Part model, mm, in its own coordinate system. A direction names the side the tool comes from. Round coordinates to 2 decimals unless told otherwise and drop trailing zeros. Write each loop counter-clockwise with the first axis right and the second up, starting at its lowest first coordinate (ties: lowest second). Pieces come first, ordered by that corner, then holes.
```python
from build123d import *

# Parameters (mm, degrees)
F1_DEPTH = 12.7
F3_DEPTH = 21.336
F6_D     = 4.7625
F6_DEPTH = 3.175
F6_TIP   = 1.4307993491
F7_W     = 6.096
F7_H     = 22.606
F7_W_2   = 22.606
F7_H_2   = 6.096
F8_DEPTH = 2.54
F9_DEPTH = 2.54


with BuildPart() as f1:
    # F0 (on Top) → F1 (new body)
    with BuildSketch(Plane.XY):
        with BuildLine():
            Line((40.4105676174, 15.0449029118), (15.0105676174, 15.0449029118))
            ThreePointArc((15.0105676174, 15.0449029118), (10.5204395569, 13.1850309723), (8.6605676174, 8.6949029118))
            Line((8.6605676174, 8.6949029118), (8.6605676174, -16.7050970882))
            ThreePointArc((8.6605676174, -16.7050970882), (10.5204395569, -21.1952251488), (15.0105676174, -23.0550970882))
            Line((15.0105676174, -23.0550970882), (40.4105676174, -23.0550970882))
            ThreePointArc((40.4105676174, -23.0550970882), (44.900695678, -21.1952251488), (46.7605676174, -16.7050970882))
            Line((46.7605676174, -16.7050970882), (46.7605676174, 8.6949029118))
            ThreePointArc((46.7605676174, 8.6949029118), (44.900695678, 13.1850309723), (40.4105676174, 15.0449029118))
        make_face()
    extrude(amount=F1_DEPTH)

    # F2 (on face) → F3 (join)
    with BuildSketch(Plane.XY.offset(12.7)):
        with BuildLine():
            ThreePointArc((46.7605676174, 8.6949029118), (44.900695678, 13.1850309723), (40.4105676174, 15.0449029118))
            Line((40.4105676174, 15.0449029118), (15.0105676174, 15.0449029118))
            ThreePointArc((15.0105676174, 15.0449029118), (10.5204395569, 13.1850309723), (8.6605676174, 8.6949029118))
            Line((8.6605676174, 8.6949029118), (8.6605676174, -16.7050970882))
            ThreePointArc((8.6605676174, -16.7050970882), (10.5204395569, -21.1952251488), (15.0105676174, -23.0550970882))
            Line((15.0105676174, -23.0550970882), (40.4105676174, -23.0550970882))
            ThreePointArc((40.4105676174, -23.0550970882), (44.900695678, -21.1952251488), (46.7605676174, -16.7050970882))
            Line((46.7605676174, -16.7050970882), (46.7605676174, 8.6949029118))
        make_face()
        with BuildLine():
            ThreePointArc((10.2480676174, 7.1074029118), (12.1079395569, 11.5975309723), (16.5980676174, 13.4574029118))
            Line((16.5980676174, 13.4574029118), (38.8230676174, 13.4574029118))
            ThreePointArc((38.8230676174, 13.4574029118), (43.313195678, 11.5975309723), (45.1730676174, 7.1074029118))
            Line((45.1730676174, 7.1074029118), (45.1730676174, -15.1175970882))
            ThreePointArc((45.1730676174, -15.1175970882), (43.313195678, -19.6077251488), (38.8230676174, -21.4675970882))
            Line((38.8230676174, -21.4675970882), (16.5980676174, -21.4675970882))
            ThreePointArc((16.5980676174, -21.4675970882), (12.1079395569, -19.6077251488), (10.2480676174, -15.1175970882))
            Line((10.2480676174, -15.1175970882), (10.2480676174, 7.1074029118))
        make_face(mode=Mode.SUBTRACT)
    extrude(amount=-F3_DEPTH)

    # F6
    with Locations(Plane.XY.offset(12.7)):
        with Locations((16.2805676174, -15.4350970882), (39.1405676174, 7.4249029118)):
            Hole(F6_D / 2, depth=F6_DEPTH)
            with Locations((0, 0, -(F6_DEPTH + F6_TIP / 2))):  # 118° drill point
                Cone(0, F6_D / 2, F6_TIP, mode=Mode.SUBTRACT)

    # F7 (on face) → F8 (cut)
    with BuildSketch(Plane(origin=(0, 0, 0), x_dir=(1, 0, 0), z_dir=(0, 0, -1))):
        with Locations((16.1795334584, 1.2174902142)):
            Rectangle(F7_W, F7_H)
        with Locations((27.74332076, 16.611794867)):
            Rectangle(F7_W_2, F7_H_2)
        with Locations((24.0339235593, 1.2174902142)):
            Rectangle(F7_W, F7_H)
        with Locations((32.0157772671, 1.3521939175)):
            Rectangle(F7_W, F7_H)
        with Locations((39.7942726691, 1.2174902142)):
            Rectangle(F7_W, F7_H)
    extrude(amount=F8_DEPTH, mode=Mode.SUBTRACT)

    # F7 (on face) → F9 (cut)
    with BuildSketch(Plane(origin=(0, 0, 0), x_dir=(1, 0, 0), z_dir=(0, 0, -1))):
        with Locations((27.74332076, 16.611794867)):
            Rectangle(F7_W_2, F7_H_2)
        with Locations((16.1795334584, 1.2174902142)):
            Rectangle(F7_W, F7_H)
        with Locations((24.0339235593, 1.2174902142)):
            Rectangle(F7_W, F7_H)
        with Locations((32.0157772671, 1.3521939175)):
            Rectangle(F7_W, F7_H)
        with Locations((39.7942726691, 1.2174902142)):
            Rectangle(F7_W, F7_H)
    extrude(amount=-F9_DEPTH, mode=Mode.SUBTRACT)


solid = f1.part
```
Q1. Drop flat-ended pins along their axis: pin 1 (5 mm diameter, centred on x = 16.5, y = 2, fed in from -Z); pin 2 (6.5 mm diameter, centred on x = 25.5, y = -16, fed in from -Z). Give the stop position or say it passes through.
Values follow:
pin 1: stops at z = 2.54
pin 2: stops at z = 0
Q2. Which spindle directions (+Z, -Z, +X, -X, +Y, -Y) get a long thin tool onto all of the face, cutting with end or side? Do faces 4 (the flat face through (45.173, -4, -4)), 5 (the cylindrical face through (41.52, 7.53, 11.09)), 6 (the cylindrical face through (44.95, 13.135, 2.181)). Say none if no direction does.
Values follow:
face 4: -Z
face 5: +Z
face 6: +Z, -Z, +X, +Y
Q3. Cut at B-B on x = 30.5. Write the cut outline in (y, z).
Values follow:
outline: (-23.06, -8.64) - (-21.47, -8.64) - (-21.47, 0) - (-19.66, 0) - (-19.66, 2.54) - (-13.56, 2.54) - (-13.56, 0) - (-12.66, 0) - (-12.66, 2.54) - (9.95, 2.54) - (9.95, 0) - (13.46, 0) - (13.46, -8.64) - (15.04, -8.64) - (15.04, 12.7) - (-23.06, 12.7) - close
Q4. Cut at D-D on y = 4. Write the cut outline in (x, z), plus the area to 3 significant figures.
Values follow:
outline: (8.66, -8.64) - (10.25, -8.64) - (10.25, 0) - (13.13, 0) - (13.13, 2.54) - (19.23, 2.54) - (19.23, 0) - (20.99, 0) - (20.99, 2.54) - (27.08, 2.54) - (27.08, 0) - (28.97, 0) - (28.97, 2.54) - (35.06, 2.54) - (35.06, 0) - (36.75, 0) - (36.75, 2.54) - (42.84, 2.54) - (42.84, 0) - (45.17, 0) - (45.17, -8.64) - (46.76, -8.64) - (46.76, 12.7) - (8.66, 12.7) - close
area: 449 mm2
Q5. Cut at A-A on z = 7. Write the cut outline in (x, y).
Values follow:
outline: (8.66, -16.71) arc R6.35 ccw to (15.01, -23.06) - (40.41, -23.06) arc R6.35 ccw to (46.76, -16.71) - (46.76, 8.69) arc R6.35 ccw to (40.41, 15.04) - (15.01, 15.04) arc R6.35 ccw to (8.66, 8.69) - close
Q6. Mould opens along Y. For faces 1 (the cylindrical face through (10.57, 13.234, 2.181)), 2 (the flat face through (28, -23.055, 2)), 3 (the flat face through (40, -1, 2.54)) say: +Y half, -Y half, draft (parallel to the pull), parting line (faces both ways), or undercut.
Values follow:
face 1: +Y half
face 2: -Y half
face 3: undercut
Q7. Cut at C-C on z = -1.25. Write the cut outline in (x, y).
Values follow:
outline: (8.66, -16.71) arc R6.35 ccw to (15.01, -23.06) - (40.41, -23.06) arc R6.35 ccw to (46.76, -16.71) - (46.76, 8.69) arc R6.35 ccw to (40.41, 15.04) - (15.01, 15.04) arc R6.35 ccw to (8.66, 8.69) - close; hole (10.25, -15.12) arc R6.35 ccw to (16.6, -21.47) - (38.82, -21.47) arc R6.35 ccw to (45.17, -15.12) - (45.17, 7.11) arc R6.35 ccw to (38.82, 13.46) - (16.6, 13.46) arc R6.35 ccw to (10.25, 7.11) - close
Q8. Wall check: L1, parallel to Y at x = 32.5, z = 2.5; L2, parallel to X at y = -14.5, z = 2; L3, parallel to Y at x = 33, z = -2. Give the ranges that are in metal, low to high.
Values follow:
L1: y = -23.06 to -19.66, -13.56 to -12.66, 9.95 to 15.04
L2: x = 8.66 to 16.44, 39.05 to 46.76
L3: y = -23.06 to -21.47, 13.46 to 15.04
